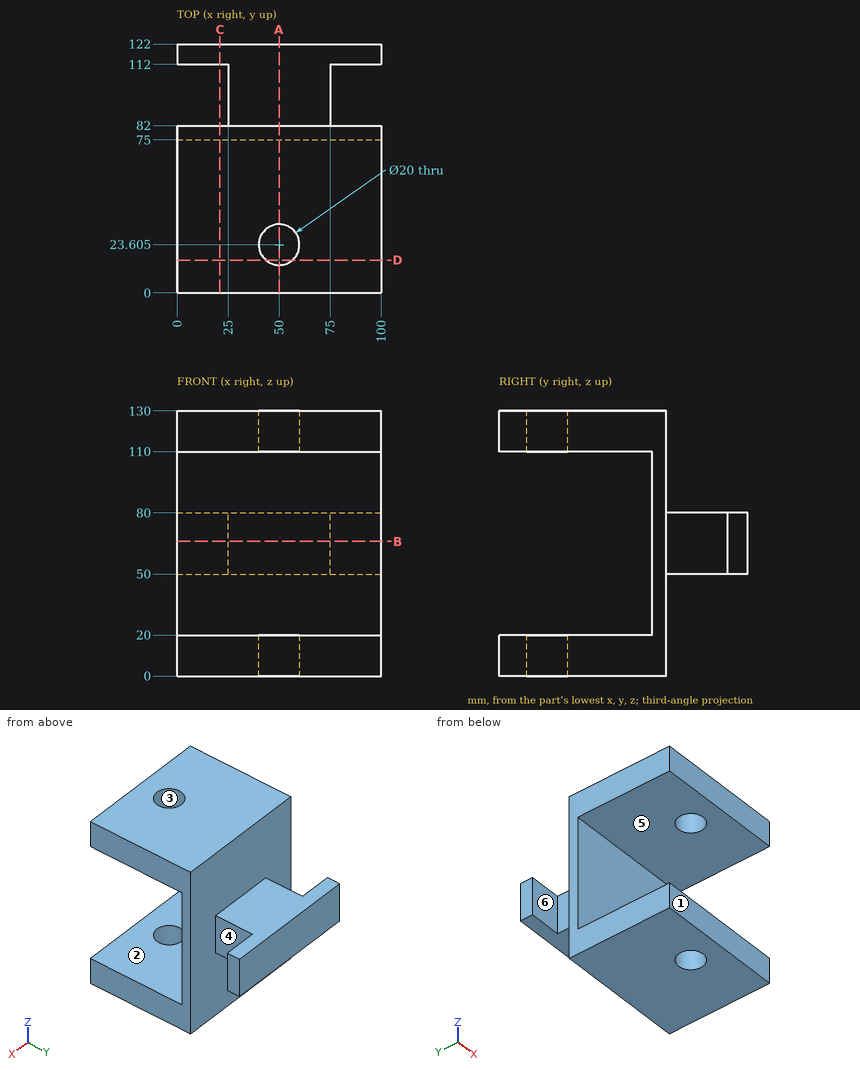
Drawing for the job (mm, zero at the part's lowest x, y, z). A direction names the side the tool comes from. Round coordinates to 2 decimals unless told otherwise and drop trailing zeros. Write each loop counter-clockwise with the first axis right and the second up, starting at its lowest first coordinate (ties: lowest second). Pieces come first, ordered by that corner, then holes. Notation, with made-up numbers: (67.5, 34) - (90.5, 34) arc R15 cw to (90.5, 49) - close; hole circle Ø4 at (-35.5, 55.5). An arc over 180 degrees is marked (long way). Return JSON: item names as keys, results as strings. Group by question number.
Item 1: Band-saw the part on C-C on x = 21. List the corners of the cut face in (y, z), plus the area to 3 significant figures.
Item 2: 3-axis set-ups, long thin cutter, end or side, ignore diameter. For the marked faces 4, 5 and 6: which of +Z, -Z, +X, -X, +Y, -Y reach the whole face in a straight line?
Item 3: Mould opens along Y. For the marked faces 1, 2 and 3 say: +Y half, -Y half, draft (parallel to the pull), parting line (faces both ways), or undercut.
Item 4: Band-saw the part on D-D on y = 16. List the corners of the cut face in (x, z).
Item 5: Probe probe 1 along Y at (x, z) = (50, 123) (1 decimal); probe 2 along Z at (x, y) = (35.5, 21); probe 3 along Y at (x, z) = (86.5, 57). List the from-to ranges inside material, lowest first.
Item 6: Band-saw the part on B-B on z = 66. List the corners of the cut face in (x, y).
Item 7: Flat gauge pins, fed straight in: pin 1 Ø12.5 at (x, z) = (84.5, 60.5) entering from -Y; pin 2 Ø15 at (y, z) = (90.5, 71) entering from +X; pin 3 Ø20 at (x, y) = (69, 93.5) entering from -Z. Where does each tip first touch, or does it go through?
Item 8: Band-saw the part on A-A on x = 50. List the corners of the cut face in (y, z) (1 decimal), plus the area to 3 significant figures.
Resolved:
{
 "1": {"outline": "(0, 0) - (82, 0) - (82, 130) - (0, 130) - (0, 110) - (75, 110) - (75, 20) - (0, 20) - close; (112, 50) - (122, 50) - (122, 80) - (112, 80) - close", "area": "4,210 mm²"},
 "2": {"face 4": "+Z, -Z, +X", "face 5": "+X, -X, -Y", "face 6": "+Z, -Z, -X"},
 "3": {"face 1": "-Y half", "face 2": "draft", "face 3": "undercut"},
 "4": {"outline": "(0, 0) - (43.51, 0) - (43.51, 20) - (0, 20) - close; (0, 110) - (43.51, 110) - (43.51, 130) - (0, 130) - close; (56.49, 0) - (100, 0) - (100, 20) - (56.49, 20) - close; (56.49, 110) - (100, 110) - (100, 130) - (56.49, 130) - close"},
 "5": {"probe 1": "y = 0 to 13.6, 33.6 to 82", "probe 2": "z = 0 to 20, 110 to 130", "probe 3": "y = 75 to 82, 112 to 122"},
 "6": {"outline": "(0, 75) - (100, 75) - (100, 82) - (75, 82) - (75, 112) - (100, 112) - (100, 122) - (0, 122) - (0, 112) - (25, 112) - (25, 82) - (0, 82) - close"},
 "7": {"pin 1": "stops at y = 75", "pin 2": "stops at x = 75", "pin 3": "stops at z = 50"},
 "8": {"outline": "(0, 0) - (13.6, 0) - (13.6, 20) - (0, 20) - close; (0, 110) - (13.6, 110) - (13.6, 130) - (0, 130) - close; (33.6, 0) - (82, 0) - (82, 50) - (122, 50) - (122, 80) - (82, 80) - (82, 130) - (33.6, 130) - (33.6, 110) - (75, 110) - (75, 20) - (33.6, 20) - close", "area": "4,310 mm²"}
}
